from build123d import *

# Parameters (mm, degrees)
F0_W     = 57
F0_H     = 57
F0_R     = 12.5
F1_DEPTH = 92
F2_DEPTH = 80
F3_DEPTH = 92.001


with BuildPart() as f1:
    # F0 (on Top) → F1 (new body)
    with BuildSketch(Plane.XY):
        Rectangle(F0_W, F0_H)
        Polygon((0, 23.5), (23.5, 23.5), (23.5, 0), (23.5, -23.5), (0, -23.5), (-23.5, -23.5), (-23.5, 0), (-23.5, 23.5), align=None, mode=Mode.SUBTRACT)
        with BuildLine():
            ThreePointArc((-23.5, 0), (-16.617009, 16.617009), (0, 23.5))
            Line((0, 23.5), (-23.5, 23.5))
            Line((-23.5, 23.5), (-23.5, 0))
        make_face()
        with BuildLine():
            Line((23.5, 0), (23.5, 23.5))
            Line((23.5, 23.5), (0, 23.5))
            ThreePointArc((0, 23.5), (16.617009, 16.617009), (23.5, 0))
        make_face()
        with BuildLine():
            Line((23.5, -23.5), (23.5, 0))
            ThreePointArc((23.5, 0), (16.617009, -16.617009), (0, -23.5))
            Line((0, -23.5), (23.5, -23.5))
        make_face()
        with BuildLine():
            ThreePointArc((0, -23.5), (-16.617009, -16.617009), (-23.5, 0))
            Line((-23.5, 0), (-23.5, -23.5))
            Line((-23.5, -23.5), (0, -23.5))
        make_face()
        with BuildLine():
            ThreePointArc((23.5, 0), (16.617009, 16.617009), (0, 23.5))
            ThreePointArc((0, 23.5), (-16.617009, 16.617009), (-23.5, 0))
            ThreePointArc((-23.5, 0), (-16.617009, -16.617009), (0, -23.5))
            ThreePointArc((0, -23.5), (16.617009, -16.617009), (23.5, 0))
        make_face()
        Circle(F0_R, mode=Mode.SUBTRACT)
        Circle(F0_R)
    extrude(amount=F1_DEPTH)

    # F0 (on Top) → F2 (cut)
    with BuildSketch(Plane.XY):
        with BuildLine():
            ThreePointArc((23.5, 0), (16.617009, 16.617009), (0, 23.5))
            ThreePointArc((0, 23.5), (-16.617009, 16.617009), (-23.5, 0))
            ThreePointArc((-23.5, 0), (-16.617009, -16.617009), (0, -23.5))
            ThreePointArc((0, -23.5), (16.617009, -16.617009), (23.5, 0))
        make_face()
        Circle(F0_R, mode=Mode.SUBTRACT)
        Circle(F0_R)
    extrude(amount=F2_DEPTH, mode=Mode.SUBTRACT)

    # F0 (on Top) → F3 (cut, through all)
    with BuildSketch(Plane.XY):
        Circle(F0_R)
    extrude(amount=F3_DEPTH, mode=Mode.SUBTRACT)


solid = f1.part
CAD build for the part. Positions are in the model's coordinates, mm. A direction names the side the tool comes from. Round coordinates to 2 decimals unless told otherwise and drop trailing zeros. Write each loop counter-clockwise with the first axis right and the second up, starting at its lowest first coordinate (ties: lowest second). Pieces come first, ordered by that corner, then holes. Notation, with made-up numbers: (-18.75, 17.5) -> (38.25, 17.5) arc R14 ccw to (38.25, 30.5) -> close; hole circle Ø10 at (-21, 44.5). An arc over 180 degrees is marked (long way). Answer as a JSON object with one key per item and string values.
(1) Band-saw the part on B-B, the plane x = -5.5. List the corners of the cut face in (y, z), then the cut area to 3 significant figures.
Reported:
{"outline": "(-28.5, 0) -> (-22.85, 0) -> (-22.85, 80) -> (-11.22, 80) -> (-11.22, 92) -> (-28.5, 92) -> close; (11.22, 80) -> (22.85, 80) -> (22.85, 0) -> (28.5, 0) -> (28.5, 92) -> (11.22, 92) -> close", "area": "1,320 mm^2"}
(2) Band-saw the part on A-A, the plane z = 73. List the corners of the cut face in (x, y).
Reported:
{"outline": "(-28.5, -28.5) -> (28.5, -28.5) -> (28.5, 28.5) -> (-28.5, 28.5) -> close; hole (-23.5, 0) arc R23.5 ccw to (0, -23.5) arc R23.5 ccw to (23.5, 0) arc R23.5 ccw to (0, 23.5) arc R23.5 ccw to start"}
(3) Band-saw the part on D-D, the plane x = -15. List the corners of the cut face in (y, z).
Reported:
{"outline": "(-28.5, 0) -> (-18.09, 0) -> (-18.09, 80) -> (18.09, 80) -> (18.09, 0) -> (28.5, 0) -> (28.5, 92) -> (-28.5, 92) -> close"}
(4) Probe probe 1 along Y at (x, z) = (0, 86); probe 2 along X at (y, z) = (-0.5, 40). List the from-to ranges inside material, lowest first. Write a range as [from, to].
Reported:
{"probe 1": "y = [-28.5, -12.5], [12.5, 28.5]", "probe 2": "x = [-28.5, -23.49], [23.49, 28.5]"}
(5) Two-plate mould, pull along Y, no slides. Class faces 1 (the face through (25, 0, 0)), 2 (the face through (11.923, 3.755, 85.916)), 3 (the face through (0, -28.5, 45)): +Y half, -Y half, draft (parallel to the pull), parting line (faces both ways), or undercut.
Reported:
{"face 1": "draft", "face 2": "undercut", "face 3": "-Y half"}
(6) Band-saw the part on C-C, the plane y = -4. List the corners of the cut face in (x, z).
Reported:
{"outline": "(-28.5, 0) -> (-23.16, 0) -> (-23.16, 80) -> (-11.84, 80) -> (-11.84, 92) -> (-28.5, 92) -> close; (11.84, 80) -> (23.16, 80) -> (23.16, 0) -> (28.5, 0) -> (28.5, 92) -> (11.84, 92) -> close"}
(7) Pin check, flat tips, straight feed: P1, Ø1.5, axis at x = -18.5, y = 17, coming from the -Z side; P2, Ø12, axis at x = 0, y = 9, coming from the -Z side. Stop position of each tip, or through.
Reported:
{"P1": "stops at z = 0", "P2": "stops at z = 80"}
(8) Which spindle directions (+Z, -Z, +X, -X, +Y, -Y) get a long thin tool onto all of the face, cutting with end or side? Do faces 4 (the face through (10, -10, 80)), 5 (the face through (28.5, 0, 45)). Say none if no direction does.
Reported:
{"face 4": "-Z", "face 5": "+Z, -Z, +X, +Y, -Y"}
